```python
from build123d import *

# Parameters (mm, degrees)
F1_ANGLE = 180
F2_T     = -2.54
F3_R     = 37.465
F3_R_2   = 36.195
F4_DEPTH = 2.54
F5_R     = 10.23543
F6_DEPTH = 101.6


with BuildPart() as f1:
    # F0 (on Top) → F1 (revolve)
    with BuildSketch(Plane.XY):
        with BuildLine():
            Line((-38.1, 0), (38.1, 0))
            ThreePointArc((38.1, 0), (0, 38.1), (-38.1, 0))
        make_face()
    revolve(axis=Axis((0, 0, 0), (1, 0, 0)), revolution_arc=F1_ANGLE)

    # F2
    f2_openings = [f1.faces().sort_by_distance(p)[0] for p in [
        (0, 0, 0),
    ]]
    offset(amount=F2_T, openings=f2_openings)

    # F3 (on Top) → F4 (cut)
    with BuildSketch(Plane.XY):
        Circle(F3_R)
        Circle(F3_R_2, mode=Mode.SUBTRACT)
    extrude(amount=F4_DEPTH, mode=Mode.SUBTRACT)

    # F5 (on Top) → F6 (cut)
    with BuildSketch(Plane.XY):
        Circle(F5_R)
    extrude(amount=F6_DEPTH, mode=Mode.SUBTRACT)


solid = f1.part
```
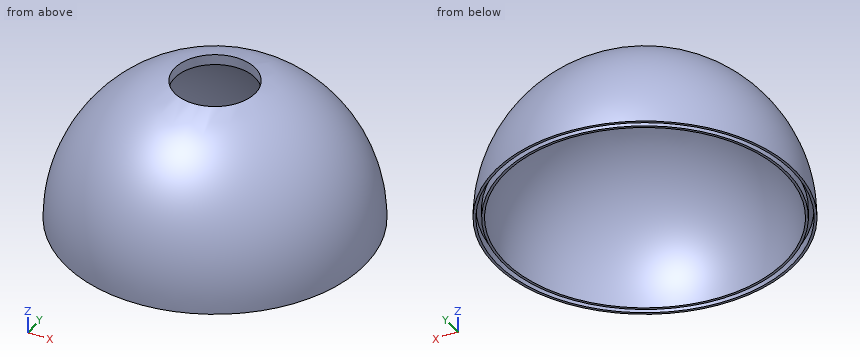
Can you work these out from the model? Positions are in its coordinate system, mm. Coordinates: 2 decimals unless noted, no trailing zeros. Order: outer loops, then holes, each group sorted by start corner. A loop starts at its lowest first (then second) coordinate and runs counter-clockwise, first axis right, second up. Notation, with made-up numbers: (84, -0.5) -> (128, -0.5) arc R20 ccw to (128, 5.5) -> close; hole circle Ø7 at (-33.75, 58.25). An arc over 180 degrees is marked (long way). Write each question's results on one line, items separated by ' | '.
Item 1: If I drill on line 1 along Y through (x, z) = (0, 1.5) (3 decimals); line 2 along X through (y, z) = (6, 2); line 3 along X through (y, z) = (-23.5, 17.5), over which ranges is the centre line in solid material (lowest first)?
Results are:
line 1: -38.07 to -37.465, -36.195 to -35.528, 35.528 to 36.195, 37.465 to 38.07 | line 2: -37.57 to -36.98, -35.69 to -34.99, 34.99 to 35.69, 36.98 to 37.57 | line 3: -24.35 to -20.15, 20.15 to 24.35
Item 2: I'm going to push flat-ended pins straight in: pin 1 Ø5 at (x, z) = (-26.5, 8) entering from +Y; pin 2 Ø4 at (x, y) = (-7.5, -18.5) entering from -Z; pin 3 Ø1 at (x, z) = (11.5, 27) entering from +Y. Where does each tip first touch, or does it pass through?
Results are:
pin 1: y = 28.59 | pin 2: z = 27.97 | pin 3: y = 24.89
Item 3: I want a section at A-A, the plane x = 0. Write out the boundary of the cut face in (y, z) (3 decimals), then the cut area to 3 significant figures.
Results are:
outline: (-38.1, 0) -> (-37.465, 0) -> (-37.465, 2.54) -> (-36.195, 2.54) -> (-36.195, 0) -> (-35.56, 0) arc R35.56 cw to (-10.235, 34.055) -> (-10.235, 36.699) arc R38.1 ccw to start; (10.235, 34.055) arc R35.56 cw to (35.56, 0) -> (36.195, 0) -> (36.195, 2.54) -> (37.465, 2.54) -> (37.465, 0) -> (38.1, 0) arc R38.1 ccw to (10.235, 36.699) -> close | area: 235 mm²
Item 4: I want a section at C-C, the plane y = 23. Write out the boundary of the cut face in (x, z), then the cut area to 3 significant figures.
Results are:
outline: (-30.37, 0) -> (-29.57, 0) -> (-29.57, 2.54) -> (-27.95, 2.54) -> (-27.95, 0) -> (-27.12, 0) arc R27.12 cw to (27.12, 0) -> (27.95, 0) -> (27.95, 2.54) -> (29.57, 2.54) -> (29.57, 0) -> (30.37, 0) arc R30.37 ccw to start | area: 286 mm²
Item 5: I want a section at D-D, the plane x = 15.5. Write out the boundary of the cut face in (y, z), then the cut area to 3 significant figures.
Results are:
outline: (-34.8, 0) -> (-34.11, 0) -> (-34.11, 2.54) -> (-32.71, 2.54) -> (-32.71, 0) -> (-32, 0) arc R32 cw to (32, 0) -> (32.71, 0) -> (32.71, 2.54) -> (34.11, 2.54) -> (34.11, 0) -> (34.8, 0) arc R34.8 ccw to start | area: 287 mm²
